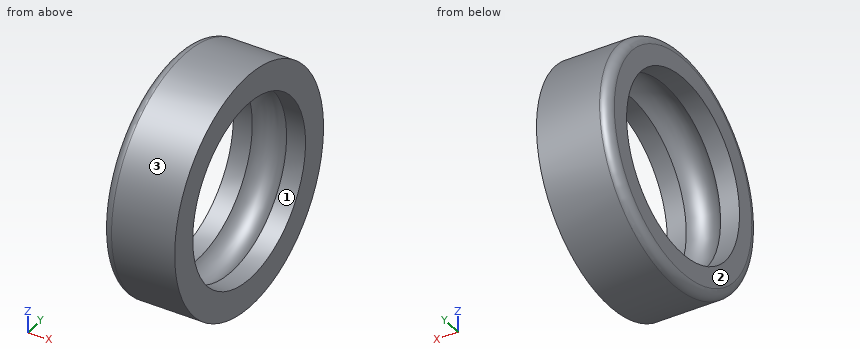
from build123d import *

# Parameters (mm, degrees)
FILLET1_R = 1


with BuildPart() as part:
    # Sketch1 → Revolve1 (revolve)
    with BuildSketch(Plane.XY, mode=Mode.PRIVATE) as revolve1_sk:
        with BuildLine():
            Line((0, 4.25), (4, 4.25))
            Line((4, 4.25), (4, 1.108))
            Line((4, 1.108), (1.900614637, 1.108))
            ThreePointArc((1.900614637, 1.108), (0, 2.2), (-1.900614637, 1.108))
            Line((-1.900614637, 1.108), (-4, 1.108))
            Line((-4, 1.108), (-4, 4.25))
            Line((-4, 4.25), (0, 4.25))
        make_face()
    revolve(revolve1_sk.sketch.rotate(Axis((4, -8.75, 0), (-1, 0, 0)), 90), axis=Axis((4, -8.75, 0), (-1, 0, 0)))

    # Fillet1
    fillet1_edges = [part.edges().sort_by_distance(p)[0] for p in [
        (-4, -8.75, 13),
    ]]
    fillet(fillet1_edges, radius=FILLET1_R)


solid = part.part
The model under review builds one solid part; all positions refer to its coordinate system, in mm. Face numbers are marked on the shaded views. Give positions to 0.01 mm unless a question says otherwise; leave off trailing zeros. Loops run counter-clockwise (first coordinate to the right, second up) from the corner with the lowest first, then second, coordinate; pieces in that order, holes last. Notation, with made-up numbers: (21.5, 3) -> (41.5, 3) arc R32 cw to (41.5, 38) -> close; hole circle Ø2 at (79, 42). An arc over 180 degrees is marked (long way). Put each result on its own line as item: value. Start each with the question number.
1. We need section B-B on y = -8.75. State the section outline as (x, z) points, then the cut area to 3 significant figures.
2. We need section A-A on z = 0. State the section outline as (x, y) points.
3. Clearance check with flat-ended pins moving along their axes: P1, Ø1.5, axis at x = -2.5, y = -5.5, coming from the -Z side; P2, Ø3, axis at x = 2, z = 9.5, coming from the -Y side. State where each tip first meets the part, or that it passes through.
4. We need section D-D on x = 1.25. State the section outline as (y, z) points.
5. Mouldability with a two-part tool opening along Y and no side actions: class the marked faces 1, 2 and 3 as released by +Y, released by -Y, zero draft, split by the parting line, or undercut.
6. We need section C-C on x = -2.5. State the section outline as (y, z) points.
7. Wall thickness on probe 1 along Y at (x, z) = (-2.6, 0); probe 2 along Y at (x, z) = (3.25, 4.75); probe 3 along Z at (x, y) = (0.25, -18.25): over which ranges is each line inside the solid? List them lowest first.
Determined:
1. outline: (-4, -12) arc R1 ccw to (-3, -13) -> (4, -13) -> (4, -9.86) -> (1.9, -9.86) arc R2.2 cw to (-1.9, -9.86) -> (-4, -9.86) -> close; (-4, 9.86) -> (-1.9, 9.86) arc R2.2 cw to (1.9, 9.86) -> (4, 9.86) -> (4, 13) -> (-3, 13) arc R1 ccw to (-4, 12) -> close
1. area: 44.0 mm^2
2. outline: (-4, -20.75) arc R1 ccw to (-3, -21.75) -> (4, -21.75) -> (4, -18.61) -> (1.9, -18.61) arc R2.2 cw to (-1.9, -18.61) -> (-4, -18.61) -> close; (-4, 1.11) -> (-1.9, 1.11) arc R2.2 cw to (1.9, 1.11) -> (4, 1.11) -> (4, 4.25) -> (-3, 4.25) arc R1 ccw to (-4, 3.25) -> close
3. P1: z = -12.76
3. P2: y = -19
4. outline: circle Ø26 at (-8.75, 0); hole circle Ø21.12 at (-8.75, 0)
5. face 1: undercut
5. face 2: zero draft
5. face 3: split by the parting line
6. outline: circle Ø26 at (-8.75, 0); hole circle Ø19.72 at (-8.75, 0)
7. probe 1: -21.75 to -18.61, 1.11 to 4.25
7. probe 2: -20.85 to -17.39, -0.11 to 3.35
7. probe 3: -8.87 to -5.42, 5.42 to 8.87
